```python
from build123d import *

# Parameters (mm, degrees)
SKETCH1_W           = 7
SKETCH1_H           = 24
BOSS_EXTRUDE1_DEPTH = 4.5
SKETCH2_W           = 7
SKETCH2_H           = 5
BOSS_EXTRUDE2_DEPTH = 0.5
SKETCH3_R           = 1.7
CUT_EXTRUDE1_DEPTH  = 57.515484604
SKETCH4_R           = 3
CUT_EXTRUDE2_DEPTH  = 2


with BuildPart() as part:
    # Sketch1 → Boss-Extrude1 (new body)
    with BuildSketch(Plane(origin=(0, 6, 0), x_dir=(1, 0, 0), z_dir=(0, 1, 0))):
        with Locations((-51.5, 0)):
            Rectangle(SKETCH1_W, SKETCH1_H)
    extrude(amount=BOSS_EXTRUDE1_DEPTH)

    # Sketch2 → Boss-Extrude2 (add)
    with BuildSketch(Plane(origin=(0, 6, 0), x_dir=(1, 0, 0), z_dir=(0, 1, 0))):
        with Locations((-51.5, 0)):
            Rectangle(SKETCH2_W, SKETCH2_H)
    extrude(amount=-BOSS_EXTRUDE2_DEPTH)

    # Sketch3 → Cut-Extrude1 (cut, through all)
    with BuildSketch(Plane(origin=(0, 10.5, 0), x_dir=(1, 0, 0), z_dir=(0, 1, 0))):
        with Locations(Location((-51.5, 7.5, 0), (0, 0, 270))):
            Circle(SKETCH3_R)
        with Locations(Location((-51.5, -7.5, 0), (0, 0, 270))):
            Circle(SKETCH3_R)
    extrude(amount=-CUT_EXTRUDE1_DEPTH, mode=Mode.SUBTRACT)

    # Sketch4 → Cut-Extrude2 (cut)
    with BuildSketch(Plane(origin=(0, 10.5, 0), x_dir=(1, 0, 0), z_dir=(0, 1, 0))):
        with Locations(Location((-51.5, 7.5, 0), (0, 0, 270))):
            Circle(SKETCH4_R)
        with Locations(Location((-51.5, -7.5, 0), (0, 0, 270))):
            Circle(SKETCH4_R)
    extrude(amount=-CUT_EXTRUDE2_DEPTH, mode=Mode.SUBTRACT)


solid = part.part
```
The listing builds one solid part. Answer for the finished solid, in the listing's coordinates (mm). A direction names the side the tool comes from. Give positions to 0.01 mm unless a question says otherwise; leave off trailing zeros. Loops run counter-clockwise (first coordinate to the right, second up) from the corner with the lowest first, then second, coordinate; pieces in that order, holes last. Notation, with made-up numbers: (88.5, 40) - (109.5, 40) arc R23 ccw to (109.5, 78) - close; hole circle Ø3 at (58.5, 10). An arc over 180 degrees is marked (long way). Answer as CSV lines item,"result". Start each with the question number.
Item 1: A cutting plane is placed at D-D on x = -50.5. Determine the outline of the cut face in (y, z), then the cut area to 3 significant figures.
Item 2: A cutting plane is placed at C-C on y = 9.2. Determine the outline of the cut face in (x, z), then the cut area to 3 significant figures.
Item 3: The mould has two halves that part along Z. Classify faces 1 (the face through (-53, 8.5, -6)), 2 (the face through (-48.97, 9.51, -5.89)), 3 (the face through (-52, 10.5, 0)), 4 (the face through (-52, 8, 12)): +Z half, -Z half, draft (parallel to the pull), parting line (faces both ways), or undercut.
Item 4: This flat-tipped pin is pushed along its axis until it touches: pin 1 (2 mm diameter, centred on x = -50, z = 9.5, fed in from -Y). Where does it stop, or does it pass through?
Item 5: A cutting plane is placed at B-B on x = -51.5. Determine the outline of the cut face in (y, z), then the cut area to 3 significant figures.
Item 6: For faces 5 (the face through (-50, 6, -6)), 6 (the face through (-53, 8.5, 9)), 7 (the face through (-53, 6, 6)), determine the directions among +Z, -Z, +X, -X, +Y, -Y from which every point of the face is accessible in a straight line to the end or side of a thin tool.
Item 7: Find the intervals of material crossed by line 1 (X direction, y = 7.35, z = -7.5); line 2 (Z direction, x = -52.75, y = 9.2); line 3 (Z direction, x = -50.75, y = 9.2), in increasing order. Write a range as from..to.
Item 8: A cutting plane is placed at A-A on z = 7.5. Determine the outline of the cut face in (x, y).
Found:
1,outline,"(5.5, -2.5) - (6, -2.5) - (6, -6.13) - (8.5, -6.13) - (8.5, -4.67) - (10.5, -4.67) - (10.5, 4.67) - (8.5, 4.67) - (8.5, 6.13) - (6, 6.13) - (6, 2.5) - (5.5, 2.5) - close; (6, -12) - (10.5, -12) - (10.5, -10.33) - (8.5, -10.33) - (8.5, -8.87) - (6, -8.87) - close; (6, 8.87) - (8.5, 8.87) - (8.5, 10.33) - (10.5, 10.33) - (10.5, 12) - (6, 12) - close"
1,area,"74.1 mm^2"
2,outline,"(-55, -12) - (-48, -12) - (-48, 12) - (-55, 12) - close; hole circle Ø6 at (-51.5, -7.5); hole circle Ø6 at (-51.5, 7.5)"
2,area,"111 mm^2"
3,face 1,"undercut"
3,face 2,"undercut"
3,face 3,"draft"
3,face 4,"+Z half"
4,pin 1,"stops at y = 6"
5,outline,"(5.5, -2.5) - (6, -2.5) - (6, -5.8) - (8.5, -5.8) - (8.5, -4.5) - (10.5, -4.5) - (10.5, 4.5) - (8.5, 4.5) - (8.5, 5.8) - (6, 5.8) - (6, 2.5) - (5.5, 2.5) - close; (6, -12) - (10.5, -12) - (10.5, -10.5) - (8.5, -10.5) - (8.5, -9.2) - (6, -9.2) - close; (6, 9.2) - (8.5, 9.2) - (8.5, 10.5) - (10.5, 10.5) - (10.5, 12) - (6, 12) - close"
5,area,"69.5 mm^2"
6,face 5,"-Z, +X, -X, -Y"
6,face 6,"+Y"
6,face 7,"+Z, +X, -X, -Y"
7,line 1,"x = -55..-53.2, -49.8..-48"
7,line 2,"z = -12..-10.23, -4.77..4.77, 10.23..12"
7,line 3,"z = -12..-10.4, -4.6..4.6, 10.4..12"
8,outline,"(-55, 6) - (-53.2, 6) - (-53.2, 8.5) - (-54.5, 8.5) - (-54.5, 10.5) - (-55, 10.5) - close; (-49.8, 6) - (-48, 6) - (-48, 10.5) - (-48.5, 10.5) - (-48.5, 8.5) - (-49.8, 8.5) - close"
